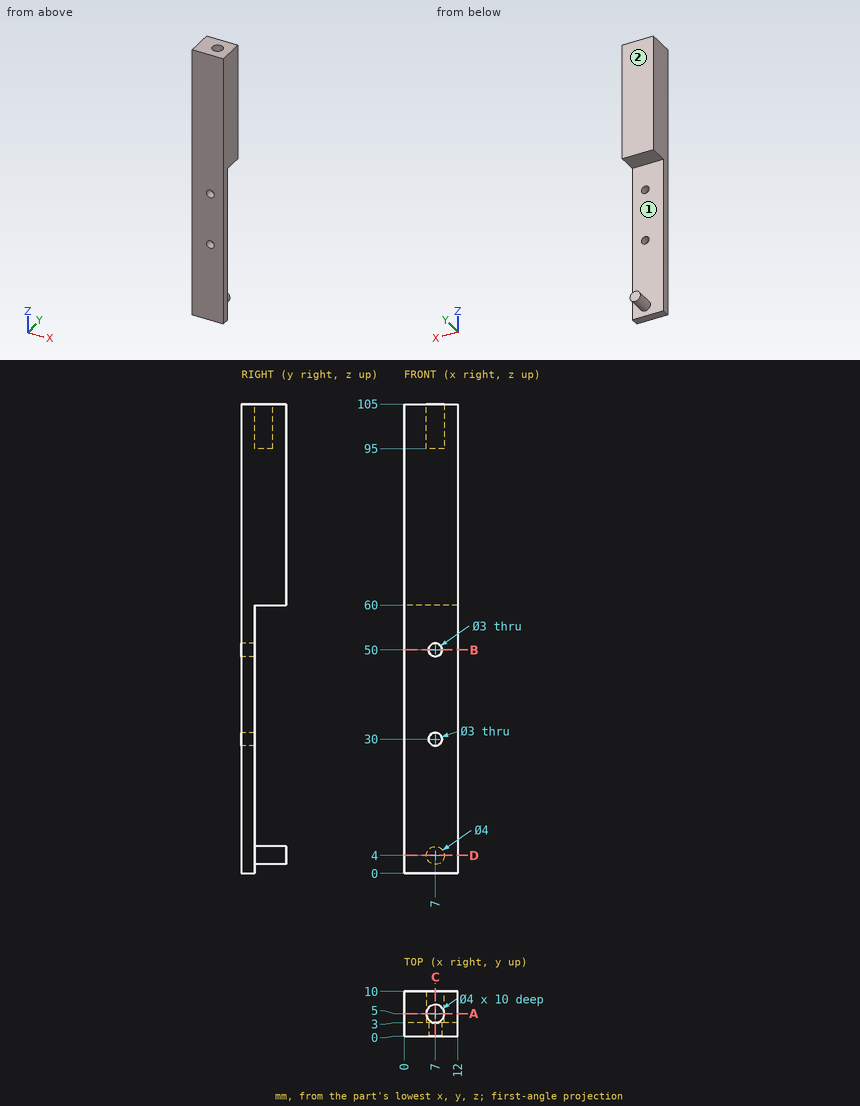
For this review, use the dimensioned drawing (mm, ordinates from the lowest corner) and the shaded views. Coordinates: 2 decimals unless noted, no trailing zeros. Loops run counter-clockwise (first coordinate to the right, second up) from the corner with the lowest first, then second, coordinate; pieces in that order, holes last. Notation, with made-up numbers: (38.5, 65.5) -> (64.5, 65.5) arc R36 cw to (64.5, 103.5) -> close; hole circle Ø1 at (80.5, -15). An arc over 180 degrees is marked (long way). Write each question's results on one line, items separated by ' | '.
Q1. Add section A-A, the plane y = 5. State the section outline as (x, z) points, then the cut area to 3 significant figures.
Taken from the geometry:
outline: (0, 60) -> (12, 60) -> (12, 105) -> (9, 105) -> (9, 95) -> (5, 95) -> (5, 105) -> (0, 105) -> close; circle Ø4 at (7, 4) | area: 513 mm²
Q2. To check wall thickness, follow line 1 along Z through (x, y) = (7, 2.2); line 2 along Y through (x, z) = (7, 102.75); line 3 along Z through (x, y) = (7, 4). State the ranges of each line that lie inside material, in increasing order. Write a range as [from, to].
Taken from the geometry:
line 1: [0, 28.5], [31.5, 48.5], [51.5, 105] | line 2: [0, 3], [7, 10] | line 3: [2, 6], [60, 95]
Q3. Add section B-B, the plane z = 50. State the section outline as (x, y) points.
Taken from the geometry:
outline: (0, 0) -> (5.5, 0) -> (5.5, 3) -> (0, 3) -> close; (8.5, 0) -> (12, 0) -> (12, 3) -> (8.5, 3) -> close
Q4. For pin 1 Ø6 at (x, y) = (5.5, 7.5) entering from -Z; pin 2 Ø2 at (x, y) = (4.5, 5.5) entering from -Z; pin 3 Ø4 at (x, z) = (7, 50) entering from +Y, all flat-tipped, find the tip position at first contact; note any pin that passes through.
Taken from the geometry:
pin 1: z = 2 | pin 2: z = 2.68 | pin 3: y = 3
Q5. Add section D-D, the plane z = 4. State the section outline as (x, y) points, then the cut area to 3 significant figures.
Taken from the geometry:
outline: (0, 0) -> (12, 0) -> (12, 3) -> (9, 3) -> (9, 10) -> (5, 10) -> (5, 3) -> (0, 3) -> close | area: 64.0 mm²
Q6. Add section C-C, the plane x = 7. State the section outline as (y, z) points.
Taken from the geometry:
outline: (0, 0) -> (3, 0) -> (3, 2) -> (10, 2) -> (10, 6) -> (3, 6) -> (3, 28.5) -> (0, 28.5) -> close; (0, 31.5) -> (3, 31.5) -> (3, 48.5) -> (0, 48.5) -> close; (0, 51.5) -> (3, 51.5) -> (3, 60) -> (10, 60) -> (10, 105) -> (7, 105) -> (7, 95) -> (3, 95) -> (3, 105) -> (0, 105) -> close
Q7. Mouldability with a two-part tool opening along Z and no side actions: class the marked faces 1 and 2 as +Z half, -Z half, draft (parallel to the pull), parting line (faces both ways), or undercut.
Taken from the geometry:
face 1: undercut | face 2: draft
